Verification items for the finished model (mm, model axes). Face numbers are marked on the shaded views. A direction names the side the tool comes from. Round coordinates to 2 decimals unless told otherwise and drop trailing zeros. Write each loop counter-clockwise with the first axis right and the second up, starting at its lowest first coordinate (ties: lowest second). Pieces come first, ordered by that corner, then holes. Notation, with made-up numbers: (7.5, 14.25) -> (60.5, 14.25) arc R30 ccw to (60.5, 47.25) -> close; hole circle Ø5 at (73, 27). An arc over 180 degrees is marked (long way). Answer as a JSON object with one key per item and string values. Group by question number.
(1) Sectioned sample at B-B on x = 0. Record the cut outline in (y, z), and give its area (3 significant figures).
(2) Draft check along Z on the marked faces 3, 4, 5 and 6. Enter one of: released by +Z, released by -Z, zero draft, split by the parting line, or undercut.
(3) Set-up check for the marked faces 1 and 2: record each of +Z, -Z, +X, -X, +Y, -Y from which the full face is reachable in a straight line by a thin tool's end or side.
(4) Sectioned sample at A-A on y = 1.7. Record the cut outline in (x, z).
(5) Scan lines: L1, parallel to Z at x = 0, y = 1.2; L2, parallel to X at y = 3.45, z = -0.6; L3, parallel to Y at x = 1.25, z = 2.55. Record each from-to range of solid material in increasing order. Write a range as from..to.
(6) Gauge pin test, flat end, axial feed: pin 1 Ø2 at (y, z) = (2, -1.5) entering from -X. Record the tip position at first contact, or that the pin passes through.
```python
from build123d import *

# Parameters (mm, degrees)
SKETCH_1_R      = 1.5
EXTRUDE_1_DEPTH = 2.3
SKETCH_2_R      = 2.25
SKETCH_2_R_2    = 1.5
EXTRUDE_2_DEPTH = 1.7
FILLET_1_R      = 0.4


with BuildPart() as part:
    # 草图1 → 凸台-拉伸1 (new body)
    with BuildSketch(Plane(origin=(0, 0, 0), x_dir=(1, 0, 0), z_dir=(0, 1, 0))):
        Polygon((3.117691454, 0), (1.558845727, 2.7), (-1.558845727, 2.7), (-3.117691454, 0), (-1.558845727, -2.7), (1.558845727, -2.7), align=None)
        Circle(SKETCH_1_R, mode=Mode.SUBTRACT)
    extrude(amount=EXTRUDE_1_DEPTH)

    # 草图2 → 凸台-拉伸2 (add)
    with BuildSketch(Plane(origin=(0, 2.3, 0), x_dir=(1, 0, 0), z_dir=(0, 1, 0))):
        Circle(SKETCH_2_R)
        Circle(SKETCH_2_R_2, mode=Mode.SUBTRACT)
    extrude(amount=EXTRUDE_2_DEPTH)

    # 圆角1
    fillet_1_edges = [part.edges().sort_by_distance(p)[0] for p in [
        (-2.25, 2.3, 0),
        (-2.25, 4, 0),
    ]]
    fillet(fillet_1_edges, radius=FILLET_1_R)


solid = part.part
```
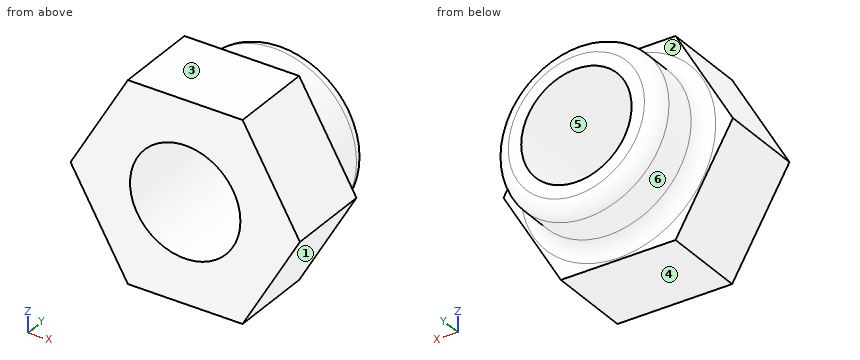
Computed values:
{
 "1": {"outline": "(0, -2.7) -> (2.3, -2.7) -> (2.3, -2.65) arc R0.4 cw to (2.7, -2.25) -> (3.6, -2.25) arc R0.4 ccw to (4, -1.85) -> (4, -1.5) -> (0, -1.5) -> close; (0, 1.5) -> (4, 1.5) -> (4, 1.85) arc R0.4 ccw to (3.6, 2.25) -> (2.7, 2.25) arc R0.4 cw to (2.3, 2.65) -> (2.3, 2.7) -> (0, 2.7) -> close", "area": "8.07 mm2"},
 "2": {"face 3": "released by +Z", "face 4": "released by -Z", "face 5": "undercut", "face 6": "split by the parting line"},
 "3": {"face 1": "-Z, +X, +Y, -Y", "face 2": "+Y"},
 "4": {"outline": "(-3.12, 0) -> (-1.56, -2.7) -> (1.56, -2.7) -> (3.12, 0) -> (1.56, 2.7) -> (-1.56, 2.7) -> close; hole circle Ø3 at (0, 0)"},
 "5": {"L1": "-2.7..-1.5, 1.5..2.7", "L2": "-2.17..-1.37, 1.37..2.17", "L3": "0..2.3"},
 "6": {"pin 1": "x = -2.83"}
}
